from build123d import *

# Parameters (mm, degrees)
F0_R     = 3
F0_R_2   = 2.5
F1_DEPTH = 490
F2_R     = 2
F3_R     = 7


# Not quite as in the source:
# - a feature names something its author has since deleted; it is built from what else it names


with BuildPart() as f1:
    # F0 (on Top) → F1 (new body)
    with BuildSketch(Plane.XY):
        with BuildLine():
            Line((18.15, -15), (30, -15))
            Line((30, -15), (30, -3.15))
            Line((30, -3.15), (27.5, -3.15))
            Line((27.5, -3.15), (27.5, -5.15))
            Line((27.5, -5.15), (21.5477069044, -5.15))
            ThreePointArc((21.5477069044, -5.15), (19.5, 0), (21.5477069044, 5.15))
            Line((21.5477069044, 5.15), (27.5, 5.15))
            Line((27.5, 5.15), (27.5, 3.15))
            Line((27.5, 3.15), (30, 3.15))
            Line((30, 3.15), (30, 15))
            Line((30, 15), (18.15, 15))
            Line((18.15, 15), (18.15, 12.5))
            Line((18.15, 12.5), (20.15, 12.5))
            Line((20.15, 12.5), (20.15, 6.5477069044))
            ThreePointArc((20.15, 6.5477069044), (15, 4.5), (9.85, 6.5477069044))
            Line((9.85, 6.5477069044), (9.85, 12.5))
            Line((9.85, 12.5), (11.85, 12.5))
            Line((11.85, 12.5), (11.85, 15))
            Line((11.85, 15), (-11.85, 15))
            Line((-11.85, 15), (-11.85, 12.5))
            Line((-11.85, 12.5), (-9.85, 12.5))
            Line((-9.85, 12.5), (-9.85, 6.5477069044))
            ThreePointArc((-9.85, 6.5477069044), (-15, 4.5), (-20.15, 6.5477069044))
            Line((-20.15, 6.5477069044), (-20.15, 12.5))
            Line((-20.15, 12.5), (-18.15, 12.5))
            Line((-18.15, 12.5), (-18.15, 15))
            Line((-18.15, 15), (-30, 15))
            Line((-30, 15), (-30, 3.15))
            Line((-30, 3.15), (-27.5, 3.15))
            Line((-27.5, 3.15), (-27.5, 5.15))
            Line((-27.5, 5.15), (-21.5477069044, 5.15))
            ThreePointArc((-21.5477069044, 5.15), (-19.5, 0), (-21.5477069044, -5.15))
            Line((-21.5477069044, -5.15), (-27.5, -5.15))
            Line((-27.5, -5.15), (-27.5, -3.15))
            Line((-27.5, -3.15), (-30, -3.15))
            Line((-30, -3.15), (-30, -15))
            Line((-30, -15), (-18.15, -15))
            Line((-18.15, -15), (-18.15, -12.5))
            Line((-18.15, -12.5), (-20.15, -12.5))
            Line((-20.15, -12.5), (-20.15, -6.5477069044))
            ThreePointArc((-20.15, -6.5477069044), (-15, -4.5), (-9.85, -6.5477069044))
            Line((-9.85, -6.5477069044), (-9.85, -12.5))
            Line((-9.85, -12.5), (-11.85, -12.5))
            Line((-11.85, -12.5), (-11.85, -15))
            Line((-11.85, -15), (11.85, -15))
            Line((11.85, -15), (11.85, -12.5))
            Line((11.85, -12.5), (9.85, -12.5))
            Line((9.85, -12.5), (9.85, -6.5477069044))
            ThreePointArc((9.85, -6.5477069044), (15, -4.5), (20.15, -6.5477069044))
            Line((20.15, -6.5477069044), (20.15, -12.5))
            Line((20.15, -12.5), (18.15, -12.5))
            Line((18.15, -12.5), (18.15, -15))
        make_face()
        with Locations((-25, -10)):
            Circle(F0_R, mode=Mode.SUBTRACT)
        with Locations((25, -10)):
            Circle(F0_R, mode=Mode.SUBTRACT)
        with Locations((-15, 0)):
            Circle(F0_R_2, mode=Mode.SUBTRACT)
        with Locations((-25, 10)):
            Circle(F0_R, mode=Mode.SUBTRACT)
        Polygon((-7, 7), (-7, 12.5), (0, 12.5), (7, 12.5), (7, 7), (10, 0), (7, -7), (7, -12.5), (0, -12.5), (-7, -12.5), (-7, -7), (-10, 0), align=None, mode=Mode.SUBTRACT)
        with Locations((15, 0)):
            Circle(F0_R_2, mode=Mode.SUBTRACT)
        with Locations((25, 10)):
            Circle(F0_R, mode=Mode.SUBTRACT)
    extrude(amount=F1_DEPTH)

    # F2
    f2_edges = [f1.edges().sort_by_distance(p)[0] for p in [
        (-7, 12.5, 245),
        (7, 12.5, 245),
    ]]
    fillet(f2_edges, radius=F2_R)

    # F3
    f3_edges = [f1.edges().sort_by_distance(p)[0] for p in [
        (-7, 7, 245),
        (-10, 0, 245),
        (7, 7, 245),
        (10, 0, 245),
    ]]
    fillet(f3_edges, radius=F3_R)


solid = f1.part
Geometry check sheet. Reference: the model listing, model coordinates, mm. A direction names the side the tool comes from. Give positions to 0.01 mm unless a question says otherwise; leave off trailing zeros. Order: outer loops, then holes, each group sorted by start corner. A loop starts at its lowest first (then second) coordinate and runs counter-clockwise, first axis right, second up. Notation, with made-up numbers: M -18,-16 L 22,-16 A33 cw 22,16 Z; hole C 49.25,-14 d2. An arc over 180 degrees is marked long. Use a Markdown table: item, result.
Item 1: Section check B-B (z = 453). State how many separate pieces and enclosed holes the cut face has, and give its area (3 significant figures).
Answers follow:
| item | result |
|---|---|
| separate pieces | 1 |
| enclosed holes | 7 |
| area | 710 mm2 |
Item 2: Depth check by flat-ended pin: P1, Ø1, axis at x = -19.5, y = -10.5, coming from the -Z side. Enter the tip coordinate at first touch or a pass-through.
Answers follow:
| item | result |
|---|---|
| P1 | passes through |
Item 3: Tool access check on faces 5 (the flat face through (0, 15, 242)), 6 (the cylindrical face through (19.5, -0.1, 241.6)). Record the directions out of +Z, -Z, +X, -X, +Y, -Y that give a thin tool (end or side, any length) a straight path to the whole face; none if there is none.
Answers follow:
| item | result |
|---|---|
| face 5 | +Z, -Z, +X, -X, +Y |
| face 6 | +Z, -Z |
Item 4: Draft check along Y on faces 1 (the flat face through (0, -12.5, 242)), 2 (the flat face through (24, -15, 242)), 3 (the flat face through (30, -9, 242)), 4 (the cylindrical face through (14.9, -4.5, 241.6)). Enter one of: +Y half, -Y half, draft (parallel to the pull), parting line (faces both ways), or undercut.
Answers follow:
| item | result |
|---|---|
| face 1 | undercut |
| face 2 | -Y half |
| face 3 | draft |
| face 4 | undercut |
Item 5: Section check A-A (x = 0). Record the cut outline in (y, z).
Answers follow:
| item | result |
|---|---|
| outline | M -15,0 L -12.5,0 L -12.5,490 L -15,490 Z; M 12.5,0 L 15,0 L 15,490 L 12.5,490 Z |
Item 6: Material ranges on line 1 along X through (y, z) = (9.25, 152); line 2 along X through (y, z) = (13.5, 285.5); line 3 along Y through (x, z) = (-25, 158), recorded low to high.
Answers follow:
| item | result |
|---|---|
| line 1 | x = -30 to -27.9, -22.1 to -20.15, -9.85 to -7, 7 to 9.85, 20.15 to 22.1, 27.9 to 30 |
| line 2 | x = -30 to -18.15, -11.85 to 11.85, 18.15 to 30 |
| line 3 | y = -15 to -13, -7 to -5.15, 5.15 to 7, 13 to 15 |
